For this review, take the finished solid that the model builds, in its own axes (mm). Coordinates: 2 decimals unless noted, no trailing zeros. Loops run counter-clockwise (first coordinate to the right, second up) from the corner with the lowest first, then second, coordinate; pieces in that order, holes last. Notation, with made-up numbers: M -20.5,39 L 24.5,39 A34 ccw 24.5,76 Z; hole C 1,-29.75 d11. An arc over 180 degrees is marked long. Write item = value, one per line.
from build123d import *

# Parameters (mm, degrees)
SKETCH1_R           = 2
BOSS_EXTRUDE3_DEPTH = 3.175
SKETCH2_R           = 2.5
CUT_EXTRUDE1_DEPTH  = 4.175
BOSS_EXTRUDE4_DEPTH = 3.175
SKETCH4_R           = 2.5
CUT_EXTRUDE2_DEPTH  = 4.175
FILLET2_R           = 5.08
FILLET3_R           = 25.4
FILLET4_R           = 5.08


with BuildPart() as part:
    # Sketch1 → Boss-Extrude3 (new body)
    with BuildSketch(Plane.XY):
        Polygon((-12.628154113, 82.464660116), (-59.28812357, -10.855278797), (-112.74974727, 44.358551699), (-42.031929204, 112.83214508), (-23.460387201, 93.651920065), align=None)
        with Locations((-20.32, 81.28)):
            Circle(SKETCH1_R, mode=Mode.SUBTRACT)
        with Locations((-60.96, 0)):
            Circle(SKETCH1_R, mode=Mode.SUBTRACT)
    extrude(amount=BOSS_EXTRUDE3_DEPTH)

    # Sketch2 → Cut-Extrude1 (cut, through all)
    with BuildSketch(Plane(origin=(0, 0, 0), x_dir=(-1, 0, 0), z_dir=(0, 0, -1))):
        with Locations((95.243542319, 33.581465441)):
            Circle(SKETCH2_R)
        with Locations((31.824813554, 94.987605576)):
            Circle(SKETCH2_R)
        with Locations((81.952877746, 46.450351765)):
            Circle(SKETCH2_R)
        with Locations((45.115478127, 82.118719252)):
            Circle(SKETCH2_R)
        with Locations((56.064112078, 71.517539384)):
            Circle(SKETCH2_R)
        with Locations((69.354776651, 58.64865306)):
            Circle(SKETCH2_R)
    extrude(amount=-CUT_EXTRUDE1_DEPTH, mode=Mode.SUBTRACT)

    # Sketch3 → Boss-Extrude4 (add)
    with BuildSketch(Plane(origin=(0, 0, 0), x_dir=(-1, 0, 0), z_dir=(0, 0, -1))):
        Polygon((112.74974727, 44.358551699), (137.38417366, 20.505896995), (115.298382267, -2.30375707), (90.663955877, 21.548897635), align=None)
    extrude(amount=-BOSS_EXTRUDE4_DEPTH)

    # Sketch4 → Cut-Extrude2 (cut, through all)
    with BuildSketch(Plane(origin=(0, 0, 0), x_dir=(-1, 0, 0), z_dir=(0, 0, -1))):
        with Locations((106.404826903, 22.774383392)):
            Circle(SKETCH4_R)
        with Locations((119.695491476, 9.905497068)):
            Circle(SKETCH4_R)
    extrude(amount=-CUT_EXTRUDE2_DEPTH, mode=Mode.SUBTRACT)

    # Fillet2
    fillet2_edges = [part.edges().sort_by_distance(p)[0] for p in [
        (-59.28812357, -10.855278797, 1.5875),
        (-12.628154113, 82.464660116, 1.5875),
    ]]
    fillet(fillet2_edges, radius=FILLET2_R)

    # Fillet3
    fillet3_edges = [part.edges().sort_by_distance(p)[0] for p in [
        (-90.663955877, 21.548897635, 1.5875),
    ]]
    fillet(fillet3_edges, radius=FILLET3_R)

    # Fillet4
    fillet4_edges = [part.edges().sort_by_distance(p)[0] for p in [
        (-115.298382267, -2.30375707, 1.5875),
    ]]
    fillet(fillet4_edges, radius=FILLET4_R)


solid = part.part
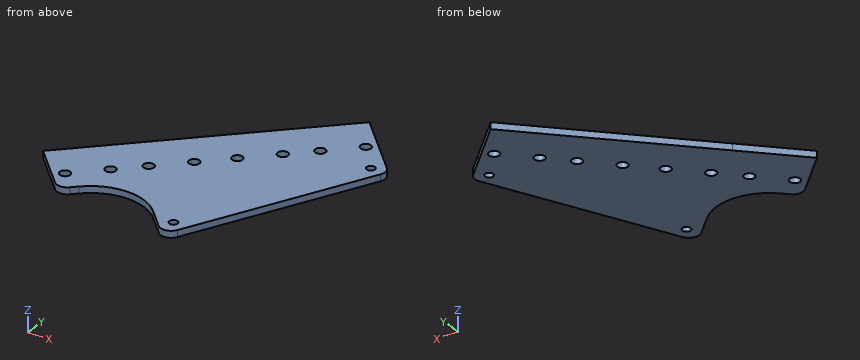
Q1. Add section A-A (x = -95). Write out the cut boundary in (y, z) (3 decimals), and give its area (3 significant figures).
Solved:
outline = M 10.753,0 L 31.093,0 L 31.093,3.175 L 10.753,3.175 Z; M 36.07,0 L 61.545,0 L 61.545,3.175 L 36.07,3.175 Z
area = 145 mm²
Q2. For line 1 along X through (y, z) = (22.5, 2.75); line 2 along Y through (x, z) = (-60.96, 2.1); line 3 along Y through (x, z) = (-20.32, 2.5), list the stretches that pass through material, from the lowest coordinate up.
Solved:
line_1 = -135.32 to -108.89, -103.92 to -42.61
line_2 = -7.24 to -2, 2 to 94.5
line_3 = 67.08 to 79.28, 83.28 to 90.41
Q3. For pin 1 Ø1.5 at (x, z) = (-47, 2.5) entering from +Y, flat-tipped, find the tip position at first contact; note if it passes through.
Solved:
pin_1 = 108.75
Q4. Add section D-D (y = 15.5). Write out the cut boundary in (x, z) (3 decimals).
Solved:
outline = M -132.537,0 L -46.11,0 L -46.11,3.175 L -132.537,3.175 Z
Q5. Add section C-C (x = -60.96). Write out the cut boundary in (y, z) (3 decimals).
Solved:
outline = M -7.24,0 L -2,0 L -2,3.175 L -7.24,3.175 Z; M 2,0 L 94.505,0 L 94.505,3.175 L 2,3.175 Z
Q6. Add section B-B (z = 0.5). State how many separate pieces and enclosed holes the cut face has, and give its area (3 significant figures).
Solved:
separate_pieces = 1
enclosed_holes = 10
area = 6,890 mm²
